from build123d import *

# Parameters (mm, degrees)
F0_W     = 127
F0_H     = 76.2
F1_DEPTH = 63.5
F2_W     = 76.2
F2_H     = 25.4
F3_DEPTH = 63.501
F4_W     = 25.4
F4_H     = 25.4
F5_DEPTH = 127.001


with BuildPart() as f1:
    # F0 (on Front) → F1 (new body)
    with BuildSketch(Plane.XZ):
        with Locations((-22.534849, -19.497559)):
            Rectangle(F0_W, F0_H)
    extrude(amount=F1_DEPTH)

    # F2 (on face) → F3 (cut, through all)
    with BuildSketch(Plane.XZ.offset(63.5)):
        with Locations((-22.534849, -44.897559)):
            Rectangle(F2_W, F2_H)
    extrude(amount=-F3_DEPTH, mode=Mode.SUBTRACT)

    # F4 (on face) → F5 (cut, through all)
    with BuildSketch(Plane.YZ.offset(40.965151)):
        with Locations((-12.7, -44.897559)):
            Rectangle(F4_W, F4_H)
        with Locations((-50.8, 5.902441)):
            Rectangle(F4_W, F4_H)
    extrude(amount=-F5_DEPTH, mode=Mode.SUBTRACT)


solid = f1.part
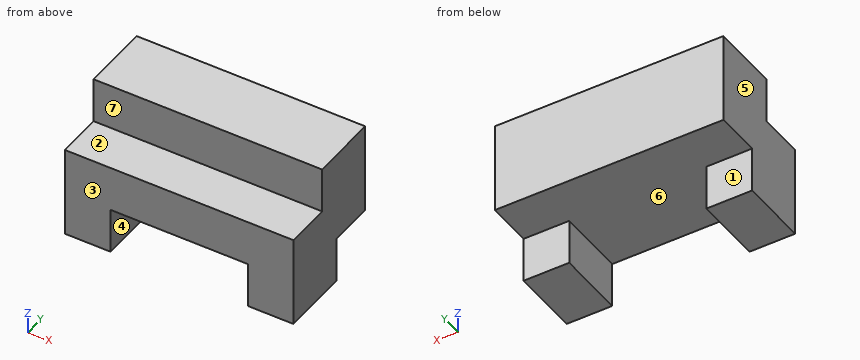
Design review of the part built by this model. Coordinates are the model's own, in mm. Face numbers are marked on the shaded views. A direction names the side the tool comes from. Round coordinates to 2 decimals unless told otherwise and drop trailing zeros. Loops run counter-clockwise (first coordinate to the right, second up) from the corner with the lowest first, then second, coordinate; pieces in that order, holes last. Notation, with made-up numbers: (61.5, -24.5) - (94.5, -24.5) arc R21 cw to (94.5, 8.5) - close; hole circle Ø6 at (23.5, 43.5). An arc over 180 degrees is marked (long way). One line per question, with ' | ' between items.
1. Draft analysis for pull direction X (two halves, no side actions). For the marked faces 5, 6 and 7, state which applies: released by +X, released by -X, zero draft, split by the parting line, or undercut.
Results are:
face 5: released by -X | face 6: undercut | face 7: zero draft
2. We need section A-A, the plane z = -36. State the section outline as (x, y) points, and give its area (3 significant figures).
Results are:
outline: (-86.03, -63.5) - (-60.63, -63.5) - (-60.63, -25.4) - (-86.03, -25.4) - close; (15.57, -63.5) - (40.97, -63.5) - (40.97, -25.4) - (15.57, -25.4) - close | area: 1,940 mm²
3. We need section B-B, the plane x = -66.5. State the section outline as (y, z) points, and give its area (3 significant figures).
Results are:
outline: (-63.5, -57.6) - (-25.4, -57.6) - (-25.4, -32.2) - (0, -32.2) - (0, 18.6) - (-38.1, 18.6) - (-38.1, -6.8) - (-63.5, -6.8) - close | area: 3,550 mm²
4. For L1, parallel to X at y = -61, z = -48.5; L2, parallel to Z at x = 31, y = -8; L3, parallel to Y at x = 8.5, z = 14, list the stretches that pass through material, from the lowest coordinate up. Write a range as [from, to].
Results are:
L1: x = [-86.03, -60.63], [15.57, 40.97] | L2: z = [-32.2, 18.6] | L3: y = [-38.1, 0]
5. We need section C-C, the plane y = -51. State the section outline as (x, z) points, and give its area (3 significant figures).
Results are:
outline: (-86.03, -57.6) - (-60.63, -57.6) - (-60.63, -32.2) - (15.57, -32.2) - (15.57, -57.6) - (40.97, -57.6) - (40.97, -6.8) - (-86.03, -6.8) - close | area: 4,520 mm²
6. Clearance check with flat-ended pins moving along their axes: P1, Ø10, axis at x = -60.5, y = -16.5, coming from the -Z side; P2, Ø10, axis at x = -63.5, z = -42, coming from the +Y side; P3, Ø20.5, axis at x = 7, z = 9, coming from the -Y side. State where each tip first meets the part, or that it passes through.
Results are:
P1: stops at z = -32.2 | P2: stops at y = -25.4 | P3: stops at y = -38.1
7. We need section D-D, the plane x = 12. State the section outline as (y, z) points.
Results are:
outline: (-63.5, -32.2) - (0, -32.2) - (0, 18.6) - (-38.1, 18.6) - (-38.1, -6.8) - (-63.5, -6.8) - close
8. For the marked faces 1, 2, 3 and 4, list the 3-axis set-ups (+Z, -Z, +X, -X, +Y, -Y) from which the entire face can be reached by the end or side of a thin tool; tool diameter is ignored.
Results are:
face 1: -Z, +X, -X, +Y | face 2: +Z, +X, -X, -Y | face 3: +Z, -Z, +X, -X, -Y | face 4: -Z, +Y, -Y
